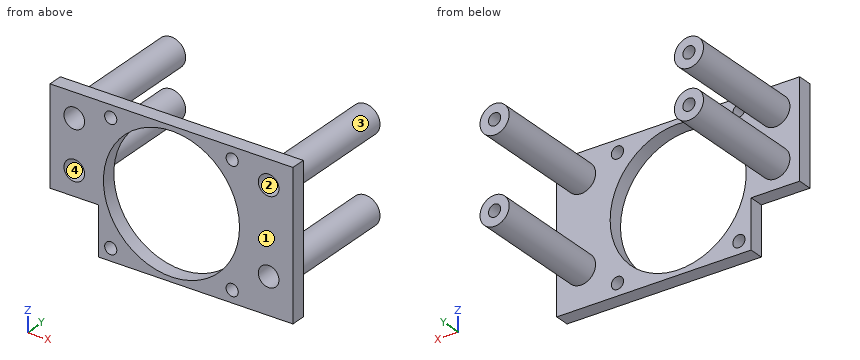
from build123d import *

# Parameters (mm, degrees)
SKETCH1_R           = 28
SKETCH1_R_2         = 2.5
BOSS_EXTRUDE1_DEPTH = 6
SKETCH2_R           = 6
BOSS_EXTRUDE2_DEPTH = 50
SKETCH3_R           = 2.5
CUT_EXTRUDE1_DEPTH  = 57
SKETCH5_R           = 4.25
CUT_EXTRUDE2_DEPTH  = 50


with BuildPart() as part:
    # Sketch1 → Boss-Extrude1 (new body)
    with BuildSketch(Plane(origin=(0, 0, 0), x_dir=(1, 0, 0), z_dir=(0, 1, 0))):
        Polygon((-50, -30), (50, -30), (50, 30), (-30, 30), (-30, 10), (-50, 10), align=None)
        Circle(SKETCH1_R, mode=Mode.SUBTRACT)
        with Locations((-25, 25)):
            Circle(SKETCH1_R_2, mode=Mode.SUBTRACT)
        with Locations((25, 25)):
            Circle(SKETCH1_R_2, mode=Mode.SUBTRACT)
        with Locations((25, -25)):
            Circle(SKETCH1_R_2, mode=Mode.SUBTRACT)
        with Locations((-25, -25)):
            Circle(SKETCH1_R_2, mode=Mode.SUBTRACT)
    extrude(amount=BOSS_EXTRUDE1_DEPTH)

    # Sketch2 → Boss-Extrude2 (add)
    with BuildSketch(Plane(origin=(0, 6, 0), x_dir=(1, 0, 0), z_dir=(0, 1, 0))):
        with Locations((-40, 0)):
            Circle(SKETCH2_R)
        with Locations((-40, -20)):
            Circle(SKETCH2_R)
        with Locations((40, 15)):
            Circle(SKETCH2_R)
        with Locations((40, -20)):
            Circle(SKETCH2_R)
    extrude(amount=BOSS_EXTRUDE2_DEPTH)

    # Sketch3 → Cut-Extrude1 (cut, through all)
    with BuildSketch(Plane(origin=(0, 56, 0), x_dir=(1, 0, 0), z_dir=(0, 1, 0))):
        with Locations((-40, 0)):
            Circle(SKETCH3_R)
        with Locations((-40, -20)):
            Circle(SKETCH3_R)
        with Locations((40, -20)):
            Circle(SKETCH3_R)
        with Locations((40, 15)):
            Circle(SKETCH3_R)
    extrude(amount=-CUT_EXTRUDE1_DEPTH, mode=Mode.SUBTRACT)

    # Sketch5 → Cut-Extrude2 (cut)
    with BuildSketch(Plane.XZ):
        with Locations((-40, 0)):
            Circle(SKETCH5_R)
        with Locations((-40, 20)):
            Circle(SKETCH5_R)
        with Locations((40, 20)):
            Circle(SKETCH5_R)
        with Locations((40, -15)):
            Circle(SKETCH5_R)
    extrude(amount=-CUT_EXTRUDE2_DEPTH, mode=Mode.SUBTRACT)


solid = part.part
Design review of the part built by this model. Coordinates are the model's own, in mm. Face numbers are marked on the shaded views. A direction names the side the tool comes from. Give positions to 0.01 mm unless a question says otherwise; leave off trailing zeros. Write each loop counter-clockwise with the first axis right and the second up, starting at its lowest first coordinate (ties: lowest second). Pieces come first, ordered by that corner, then holes. Notation, with made-up numbers: M -29,-1 L -9,-1 A18 ccw -9,33 Z; hole C 10.25,28 d7. An arc over 180 degrees is marked long. Answer as a JSON object with one key per item and string values. Group by question number.
1) We need section A-A (y = 31). Give the boundary of the cut face in (x, z).
2) We need section C-C (x = 40). Give the boundary of the cut face in (y, z), and give its area (3 significant figures).
3) We need section B-B (x = 0). Give the boundary of the cut face in (y, z), and give its area (3 significant figures).
4) Tool access review of the marked faces 3 and 4: name each direction out of +Z, -Z, +X, -X, +Y, -Y from which nothing blocks a thin tool from reaching the whole face with its end or side.
5) Clearance check with flat-ended pins moving along their axes: pin 1 Ø3 at (x, z) = (-40, 0) entering from -Y; pin 2 Ø6 at (y, z) = (26, 17.5) entering from +X; pin 3 Ø6.5 at (x, y) = (-38.5, 3) entering from -Z; pin 4 Ø4 at (x, z) = (-32.5, -6.5) entering from +Y. State where each tip first meets the part, or that it passes through.
6) Mouldability with a two-part tool opening along Z and no side actions: class the marked faces 1 and 2 as released by +Z, released by -Z, zero draft, split by the parting line, or undercut.
7) We need section D-D (z = -15). Give the boundary of the cut face in (x, y).
8) For line 1 along Z through (x, y) = (40, 32); line 2 along Z through (x, y) = (-40, 10.5); line 3 along X through (y, z) = (24, 21.5), list the stretches that pass through material, from the lowest coordinate up.
Answer key:
{
 "1": {"outline": "C -40,0 d12; C -40,20 d12; C 40,-15 d12; C 40,20 d12; hole C -40,0 d8.5; hole C -40,20 d8.5; hole C 40,-15 d8.5; hole C 40,20 d8.5"},
 "2": {"outline": "M 0,-30 L 6,-30 L 6,-21 L 56,-21 L 56,-17.5 L 50,-17.5 L 50,-19.25 L 0,-19.25 Z; M 0,-10.75 L 50,-10.75 L 50,-12.5 L 56,-12.5 L 56,-9 L 6,-9 L 6,14 L 56,14 L 56,17.5 L 50,17.5 L 50,15.75 L 0,15.75 Z; M 0,24.25 L 50,24.25 L 50,22.5 L 56,22.5 L 56,26 L 6,26 L 6,30 L 0,30 Z", "area": "650 mm²"},
 "3": {"outline": "M 0,-30 L 6,-30 L 6,-28 L 0,-28 Z; M 0,28 L 6,28 L 6,30 L 0,30 Z", "area": "24.0 mm²"},
 "4": {"face 3": "+Y", "face 4": "-Y"},
 "5": {"pin 1": "passes through", "pin 2": "stops at x = 46", "pin 3": "stops at z = -10", "pin 4": "stops at y = 6"},
 "6": {"face 1": "zero draft", "face 2": "undercut"},
 "7": {"outline": "M -30,0 L -23.64,0 L -23.64,6 L -30,6 Z; M 23.64,0 L 35.75,0 L 35.75,50 L 37.5,50 L 37.5,56 L 34,56 L 34,6 L 23.64,6 Z; M 42.5,50 L 44.25,50 L 44.25,0 L 50,0 L 50,6 L 46,6 L 46,56 L 42.5,56 Z"},
 "8": {"line 1": "z = -21 to -19.25, -10.75 to -9, 14 to 15.75, 24.25 to 26", "line 2": "z = -6 to -4.25, 4.25 to 6, 14 to 15.75, 24.25 to 26", "line 3": "x = -45.81 to -43.98, -36.02 to -34.19, 34.19 to 36.02, 43.98 to 45.81"}
}
